Can you work these out from the drawing? Everything is in mm from the part's minimum corner. A direction names the side the tool comes from. Coordinates: 2 decimals unless noted, no trailing zeros. Order: outer loops, then holes, each group sorted by start corner. A loop starts at its lowest first (then second) coordinate and runs counter-clockwise, first axis right, second up. Notation, with made-up numbers: (4, 42) -> (24, 42) arc R15 ccw to (24, 55) -> close; hole circle Ø7 at (-25.5, 70.5). An arc over 180 degrees is marked (long way). Write item = value, one per line. Start each with the question number.
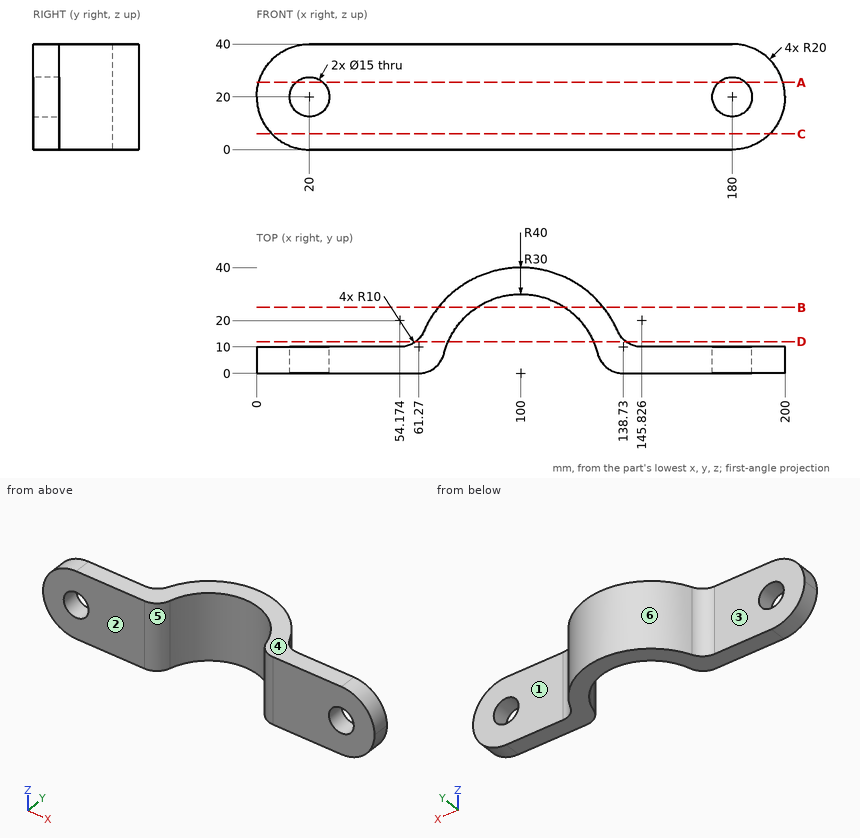
(1) Imagine slicing it at B-B (y = 25). Write out the boundary of the cut face in (x, z) (1 decimal).
(2) For P1, Ø8, axis at y = 12, z = 6, coming from the -X side; P2, Ø9, axis at x = 20, z = 20, coming from the +Y side; P3, Ø1, axis at x = 77, z = 11, coming from the +Y side; P4, Ø20, axis at x = 20.5, z = 21, coming from the +Y side, each with a flat end and sliding along its axis, tell me the tip position at first contact or that it passes through.
(3) If I drill on L1, parallel to X at y = 3.5, z = 20; L2, parallel to X at y = 5.75, z = 20; L3, parallel to Y at x = 170.5, z = 17, over which ranges is the centre line in solid material (lowest first)? Write a range as from..to.
(4) Thinking about a two-plate mould opening in X: for the marked faces 4, 5 and 6, which applies, +X half, -X half, draft (parallel to the pull), parting line (faces both ways), or undercut?
(5) Imagine slicing it at C-C (z = 6). Write out the boundary of the cut face in (x, y).
(6) Imagine slicing it at D-D (y = 12). Write out the boundary of the cut face in (x, z) (1 decimal).
(7) For the marked faces 1, 2 and 3, which set-ups out of +Z, -Z, +X, -X, +Y, -Y let a thin tool reach every point of the face, with its end or its side?
(8) Imagine slicing it at A-A (z = 25.5). Write out the boundary of the cut face in (x, y).
Result set:
q1.outline = (68.8, 0) -> (83.4, 0) -> (83.4, 40) -> (68.8, 40) -> close; (116.6, 0) -> (131.2, 0) -> (131.2, 40) -> (116.6, 40) -> close
q2.P1 = 3
q2.P2 = through
q2.P3 = 33.07
q2.P4 = 10
q3.L1 = 0..12.5, 27.5..68.87, 131.13..172.5, 187.5..200
q3.L2 = 0..12.5, 27.5..70.32, 129.68..172.5, 187.5..200
q3.L3 = 0..10
q4.face_4 = draft
q4.face_5 = undercut
q4.face_6 = parting line
q5.outline = (5.72, 0) -> (61.27, 0) arc R10 ccw to (70.95, 7.5) arc R30 cw to (129.05, 7.5) arc R10 ccw to (138.73, 0) -> (194.28, 0) -> (194.28, 10) -> (145.83, 10) arc R10 cw to (136.66, 16) arc R40 ccw to (63.34, 16) arc R10 cw to (54.17, 10) -> (5.72, 10) -> close
q6.outline = (60.2, 0) -> (72.5, 0) -> (72.5, 40) -> (60.2, 40) -> close; (127.5, 0) -> (139.8, 0) -> (139.8, 40) -> (127.5, 40) -> close
q7.face_1 = +Z, -Z, +X, +Y
q7.face_2 = +Z, -Z, +X, -X, -Y
q7.face_3 = +Z, -Z, -X, +Y
q8.outline = (0.77, 0) -> (14.9, 0) -> (14.9, 10) -> (0.77, 10) -> close; (25.1, 0) -> (61.27, 0) arc R10 ccw to (70.95, 7.5) arc R30 cw to (129.05, 7.5) arc R10 ccw to (138.73, 0) -> (174.9, 0) -> (174.9, 10) -> (145.83, 10) arc R10 cw to (136.66, 16) arc R40 ccw to (63.34, 16) arc R10 cw to (54.17, 10) -> (25.1, 10) -> close; (185.1, 0) -> (199.23, 0) -> (199.23, 10) -> (185.1, 10) -> close
